```python
from build123d import *

# Parameters (mm, degrees)
F1_DEPTH = 15
F2_W     = 3
F2_H     = 15
F3_DEPTH = 6
F4_R     = 2.25
F5_DEPTH = 25
F6_R     = 0.5
F7_R     = 0.5


with BuildPart() as f1:
    # F0 (on Front) → F1 (new body)
    with BuildSketch(Plane.XZ):
        with BuildLine():
            ThreePointArc((4.2, 0), (0, -4.2), (-4.2, 0))
            Line((-4.2, 0), (-7.2, 0))
            Line((-7.2, 0), (-7.2, -10.624883))
            Line((-7.2, -10.624883), (16.2, -10.624883))
            Line((16.2, -10.624883), (16.2, -6.216642))
            Line((16.2, -6.216642), (7.2, -6.216642))
            Line((7.2, -6.216642), (7.2, 0))
            Line((7.2, 0), (4.2, 0))
        make_face()
    extrude(amount=F1_DEPTH)

    # F2 (on face) → F3 (join)
    with BuildSketch(Plane.XY):
        with Locations((-5.7, -7.5)):
            Rectangle(F2_W, F2_H)
        with Locations((5.7, -7.5)):
            Rectangle(F2_W, F2_H)
    extrude(amount=F3_DEPTH)

    # F4 (on face) → F5 (cut)
    with BuildSketch(Plane.XY.offset(-6.216642)):
        with Locations((11.7, -7.5)):
            Circle(F4_R)
    extrude(amount=-F5_DEPTH, mode=Mode.SUBTRACT)

    # F6
    f6_edges = [f1.edges().sort_by_distance(p)[0] for p in [
        (-7.2, -7.5, -10.624883),
        (16.2, -7.5, -10.624883),
        (-7.2, -7.5, 6),
        (-4.2, -7.5, 6),
        (4.2, -7.5, 6),
        (7.2, -7.5, 6),
        (7.2, -7.5, -6.216642),
    ]]
    fillet(f6_edges, radius=F6_R)

    # F7
    f7_edges = [f1.edges().sort_by_distance(p)[0] for p in [
        (16.2, -7.5, -6.216642),
    ]]
    fillet(f7_edges, radius=F7_R)


solid = f1.part
```
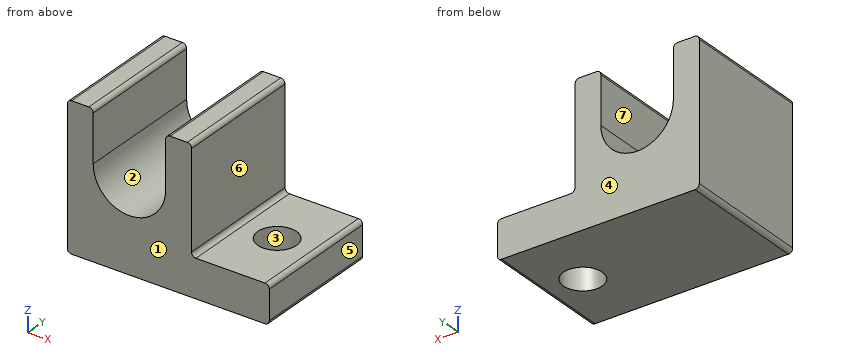
The listing builds one solid part. Answer for the finished solid, in the listing's coordinates (mm). Face numbers are marked on the shaded views. A direction names the side the tool comes from. Coordinates: 2 decimals unless noted, no trailing zeros. Write each loop counter-clockwise with the first axis right and the second up, starting at its lowest first coordinate (ties: lowest second). Pieces come first, ordered by that corner, then holes. Notation, with made-up numbers: (25.25, 22.25) -> (55.25, 22.25) arc R30 ccw to (55.25, 48.25) -> close; hole circle Ø3 at (4.25, 16.25). An arc over 180 degrees is marked (long way). Write each question's results on one line, items separated by ' | '. Start each with the question number.
1) Flat-ended cylindrical pins translate along their axes: pin 1 Ø1 at (y, z) = (-8.5, -5.5) entering from +X; pin 2 Ø6 at (x, z) = (2.5, -2.5) entering from +Y; pin 3 Ø1 at (y, z) = (-11.5, -2) entering from +X; pin 4 Ø6 at (x, y) = (11.7, -7.5) entering from +Z. Find the tip coordinate at first contact, or state that the pin passes through.
2) A cutting plane is placed at B-B (x = 11.7). Determine the outline of the cut face in (y, z).
3) For a pull along Y with two mould halves and no side action, classify the marked faces 1, 2, 3 and 4 as +Y half, -Y half, draft (parallel to the pull), parting line (faces both ways), or undercut.
4) A cutting plane is placed at A-A (y = -7.5). Determine the outline of the cut face in (x, z), then the cut area to 3 significant figures.
5) Straight lines are drawn through the part: probe 1 along Y at (x, z) = (11.7, -9.3); probe 2 along X at (y, z) = (-7.5, 3.75); probe 3 along X at (y, z) = (-9.25, -5.75). For each, find the intervals that lie inside material, in ascending order.
6) A cutting plane is placed at C-C (z = -7.25). Determine the outline of the cut face in (x, y).
7) A tool of negligible diameter and unlimited length cuts with its end or side. For the marked faces 5, 6 and 7, from which of +Z, -Z, +X, -X, +Y, -Y can it reach the whole face along a straight path? Write none if from no direction.
8) A cutting plane is placed at D-D (y = -4.5). Determine the outline of the cut face in (x, z).
Values follow:
1) pin 1: x = 7.29 | pin 2: y = 0 | pin 3: x = 7.2 | pin 4: z = -6.22
2) outline: (-15, -10.62) -> (-9.75, -10.62) -> (-9.75, -6.22) -> (-15, -6.22) -> close; (-5.25, -10.62) -> (0, -10.62) -> (0, -6.22) -> (-5.25, -6.22) -> close
3) face 1: -Y half | face 2: draft | face 3: undercut | face 4: +Y half
4) outline: (-7.2, -10.12) arc R0.5 ccw to (-6.7, -10.62) -> (9.45, -10.62) -> (9.45, -6.22) -> (7.7, -6.22) arc R0.5 cw to (7.2, -5.72) -> (7.2, 5.5) arc R0.5 ccw to (6.7, 6) -> (4.7, 6) arc R0.5 ccw to (4.2, 5.5) -> (4.2, 0) arc R4.2 cw to (-4.2, 0) -> (-4.2, 5.5) arc R0.5 ccw to (-4.7, 6) -> (-6.7, 6) arc R0.5 ccw to (-7.2, 5.5) -> close; (13.95, -10.62) -> (15.7, -10.62) arc R0.5 ccw to (16.2, -10.12) -> (16.2, -6.72) arc R0.5 ccw to (15.7, -6.22) -> (13.95, -6.22) -> close | area: 181 mm²
5) probe 1: -15 to -9.75, -5.25 to 0 | probe 2: -7.2 to -4.2, 4.2 to 7.2 | probe 3: -7.2 to 7.2
6) outline: (-7.2, -15) -> (16.2, -15) -> (16.2, 0) -> (-7.2, 0) -> close; hole circle Ø4.5 at (11.7, -7.5)
7) face 5: +Z, -Z, +X, +Y, -Y | face 6: +Z, +X, +Y, -Y | face 7: +Z, +Y, -Y
8) outline: (-7.2, -10.12) arc R0.5 ccw to (-6.7, -10.62) -> (15.7, -10.62) arc R0.5 ccw to (16.2, -10.12) -> (16.2, -6.72) arc R0.5 ccw to (15.7, -6.22) -> (7.7, -6.22) arc R0.5 cw to (7.2, -5.72) -> (7.2, 5.5) arc R0.5 ccw to (6.7, 6) -> (4.7, 6) arc R0.5 ccw to (4.2, 5.5) -> (4.2, 0) arc R4.2 cw to (-4.2, 0) -> (-4.2, 5.5) arc R0.5 ccw to (-4.7, 6) -> (-6.7, 6) arc R0.5 ccw to (-7.2, 5.5) -> close
